Design review of the part built by this model. Coordinates are the model's own, in mm. Face numbers are marked on the shaded views. Round coordinates to 2 decimals unless told otherwise and drop trailing zeros. Order: outer loops, then holes, each group sorted by start corner. A loop starts at its lowest first (then second) coordinate and runs counter-clockwise, first axis right, second up. Notation, with made-up numbers: (-2.5, 74.5) - (51.5, 74.5) arc R7 ccw to (51.5, 81.5) - close; hole circle Ø7 at (86.25, 0.5). An arc over 180 degrees is marked (long way). Use CSV: the item, a comma, the result in double quotes.
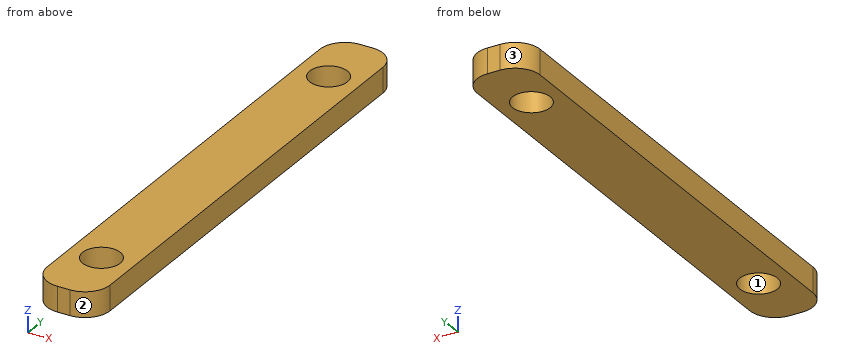
Autodesk Inventor part; units mm, degrees
ref_plane "YZ Plane" through (0, 0, 0) normal (1, 0, 0) x (0, 1, 0)
ref_plane "XZ Plane" through (0, 0, 0) normal (0, 1, 0) x (-1, 0, 0)
ref_plane "XY Plane" through (0, 0, 0) normal (0, 0, 1) x (1, 0, 0)
sketch "Skizze1" plane through (0, 0, 0) normal (0, 0, 1) x (1, 0, 0)
  line L0 (2, 26) -> (3, 26)
  line L1 (5, 28) -> (5, 64)
  line L2 (3, 66) -> (2, 66)
  line L3 (0, 64) -> (0, 28)
  arc A0 (5, 64) -> (3, 66) centre (3, 64) ccw
  arc A1 (3, 26) -> (5, 28) centre (3, 28) ccw
  arc A2 (0, 28) -> (2, 26) centre (2, 28) ccw
  arc A3 (2, 66) -> (0, 64) centre (2, 64) ccw
  point P0 (0, 0)
  point P1 (0, 26)
  point P2 (5, 66)
  point P3 (5, 26)
  point P4 (0, 66)
  dimension "d0" = 5
  dimension "d1" = 40
  dimension "d2" = 2
extrude "Extrusion1" add sketch "Skizze1" along normal blind 2
hole "Bohrung1" at (2.5, 61, 2) direction (0, 0, -1) diameter 3 end through all
hole "Bohrung2" at (2.5, 31, 2) direction (0, 0, -1) diameter 3 end through all
properties part number "Halter_Verschraubung"
1) We need section C-C (z = 1.6). Give the boundary of the cut face in (x, y), then the cut area to 3 significant figures.
Data:
outline,"(0, 28) arc R2 ccw to (2, 26) - (3, 26) arc R2 ccw to (5, 28) - (5, 64) arc R2 ccw to (3, 66) - (2, 66) arc R2 ccw to (0, 64) - close; hole circle Ø3 at (2.5, 31); hole circle Ø3 at (2.5, 61)"
area,"182 mm2"
2) We need section A-A (x = 2.5). Give the boundary of the cut face in (y, z), then the cut area to 3 significant figures.
Data:
outline,"(26, 0) - (29.5, 0) - (29.5, 2) - (26, 2) - close; (32.5, 0) - (59.5, 0) - (59.5, 2) - (32.5, 2) - close; (62.5, 0) - (66, 0) - (66, 2) - (62.5, 2) - close"
area,"68.0 mm2"
3) We need section D-D (x = 0.5). Give the boundary of the cut face in (y, z), then the cut area to 3 significant figures.
Data:
outline,"(26.68, 0) - (65.32, 0) - (65.32, 2) - (26.68, 2) - close"
area,"77.3 mm2"
4) We need section B-B (y = 61). Give the boundary of the cut face in (x, z), then the cut area to 3 significant figures.
Data:
outline,"(0, 0) - (1, 0) - (1, 2) - (0, 2) - close; (4, 0) - (5, 0) - (5, 2) - (4, 2) - close"
area,"4.00 mm2"
5) The part is to be moulded in two halves that separate along X. For the marked faces 1, 2 and 3, say which applies: +X half, -X half, draft (parallel to the pull), parting line (faces both ways), or undercut.
Data:
face 1,"undercut"
face 2,"+X half"
face 3,"-X half"
6) To check wall thickness, follow L1, parallel to Y at x = 2.5, z = 1.15; L2, parallel to X at y = 61, z = 1.1; L3, parallel to X at y = 62, z = 1.3. State the ranges of each line that lie inside material, in increasing order. Write a range as from..to.
Data:
L1,"y = 26..29.5, 32.5..59.5, 62.5..66"
L2,"x = 0..1, 4..5"
L3,"x = 0..1.38, 3.62..5"
